```python
from build123d import *

# Parameters (mm, degrees)
SKETCH1_R           = 53.975
SKETCH1_R_2         = 3.302
BOSS_EXTRUDE1_DEPTH = 3.175
SKETCH2_R           = 28.575
BOSS_EXTRUDE2_DEPTH = 136.525
SKETCH3_W           = 40.450959828
SKETCH3_H           = 34.29
CUT_EXTRUDE1_DEPTH  = 136.525
SKETCH4_W           = 24.671855952
SKETCH4_H           = 34.29
CUT_EXTRUDE2_DEPTH  = 49.53
FILLET1_R           = 2.54


with BuildPart() as part:
    # Sketch1 → Boss-Extrude1 (new body)
    with BuildSketch(Plane(origin=(0, 0, 0), x_dir=(1, 0, 0), z_dir=(0, 1, 0))):
        with Locations(Location((0, 0, 0), (0, 0, 270))):
            Circle(SKETCH1_R)
        with Locations(Location((0, 47.625, 0), (0, 0, 270))):
            Circle(SKETCH1_R_2, mode=Mode.SUBTRACT)
        with Locations(Location((45.294066589, 14.716934357, 0), (0, 0, 270))):
            Circle(SKETCH1_R_2, mode=Mode.SUBTRACT)
        with Locations(Location((27.99327264, -38.529434357, 0), (0, 0, 270))):
            Circle(SKETCH1_R_2, mode=Mode.SUBTRACT)
        with Locations(Location((-27.99327264, -38.529434357, 0), (0, 0, 270))):
            Circle(SKETCH1_R_2, mode=Mode.SUBTRACT)
        with Locations(Location((-45.294066589, 14.716934357, 0), (0, 0, 270))):
            Circle(SKETCH1_R_2, mode=Mode.SUBTRACT)
    extrude(amount=BOSS_EXTRUDE1_DEPTH)

    # Sketch2 → Boss-Extrude2 (add)
    with BuildSketch(Plane(origin=(0, 3.175, 0), x_dir=(1, 0, 0), z_dir=(0, 1, 0))):
        with Locations(Location((0, 0, 0), (0, 0, 270))):
            Circle(SKETCH2_R)
    extrude(amount=BOSS_EXTRUDE2_DEPTH)

    # Sketch3 → Cut-Extrude1 (cut)
    with BuildSketch(Plane(origin=(0, 139.7, 0), x_dir=(1, 0, 0), z_dir=(0, 1, 0))):
        with Locations((43.085479914, 0)):
            Rectangle(SKETCH3_W, SKETCH3_H)
    extrude(amount=-CUT_EXTRUDE1_DEPTH, mode=Mode.SUBTRACT)

    # Sketch4 → Cut-Extrude2 (cut)
    with BuildSketch(Plane(origin=(0, 3.175, 0), x_dir=(1, 0, 0), z_dir=(0, 1, 0))):
        with Locations((-35.195927976, 0)):
            Rectangle(SKETCH4_W, SKETCH4_H)
    extrude(amount=CUT_EXTRUDE2_DEPTH, mode=Mode.SUBTRACT)

    # Fillet1
    fillet1_edges = [part.edges().sort_by_distance(p)[0] for p in [
        (-28.575, 139.7, 0),
        (22.86, 139.7, 0),
        (22.86, 71.4375, 17.145),
        (22.86, 71.4375, -17.145),
        (-28.575, 52.705, 0),
        (-22.86, 27.94, 17.145),
        (-22.86, 27.94, -17.145),
    ]]
    fillet(fillet1_edges, radius=FILLET1_R)
    fillet1_2_edges = [part.edges().sort_by_distance(p)[0] for p in [
        (0, 3.175, -28.575),
        (22.86, 3.175, 0),
        (0, 3.175, 28.575),
        (-22.86, 3.175, 0),
        (-22.716559526, 3.175, -17.117815364),
        (-22.716559526, 3.175, 17.117815364),
        (22.716559526, 3.175, 17.117815364),
        (22.716559526, 3.175, -17.117815364),
    ]]
    fillet(fillet1_2_edges, radius=FILLET1_R)


solid = part.part
```
Geometry: final body of the model. Coordinates: model frame, mm. A direction names the side the tool comes from. Coordinates: 2 decimals unless noted, no trailing zeros. Order: outer loops, then holes, each group sorted by start corner. A loop starts at its lowest first (then second) coordinate and runs counter-clockwise, first axis right, second up. Notation, with made-up numbers: (22.5, 24) -> (73.5, 24) arc R28 ccw to (73.5, 58) -> close; hole circle Ø6 at (43.5, -39.75). An arc over 180 degrees is marked (long way). Write item = value, one per line.
(1) Cut plane A-A on x = 0. Return loops of the section in (y, z) (3 decimals).
Solved:
outline = (0, -53.975) -> (3.175, -53.975) -> (3.175, -50.927) -> (0, -50.927) -> close; (0, -44.323) -> (3.175, -44.323) -> (3.175, -31.115) arc R2.54 cw to (5.715, -28.575) -> (137.16, -28.575) arc R2.54 ccw to (139.7, -26.035) -> (139.7, 26.035) arc R2.54 ccw to (137.16, 28.575) -> (5.715, 28.575) arc R2.54 cw to (3.175, 31.115) -> (3.175, 53.975) -> (0, 53.975) -> close
(2) Cut plane D-D on y = 107. Return loops of the section in (x, z) (3 decimals), plus the area to 3 significant figures.
Solved:
outline = (22.302, -17.864) arc R2.54 ccw to (22.86, -16.276) -> (22.86, 16.276) arc R2.54 ccw to (22.302, 17.864) arc R28.575 ccw (long way) to start
area = 2,430 mm²
(3) Cut plane B-B on y = 38. Return loops of the section in (x, z) (3 decimals), plus the area to 3 significant figures.
Solved:
outline = (-22.86, -16.276) arc R2.54 ccw to (-22.302, -17.864) arc R28.575 ccw to (22.302, -17.864) arc R2.54 ccw to (22.86, -16.276) -> (22.86, 16.276) arc R2.54 ccw to (22.302, 17.864) arc R28.575 ccw to (-22.302, 17.864) arc R2.54 ccw to (-22.86, 16.276) -> close
area = 2,300 mm²
(4) Pull-direction query (X, two-part tool) for faces 1 (the cylindrical face through (0.145, 1.565, -50.924)), 2 (the flat face through (22.86, 72, 0)), 3 (the cylindrical face through (-28.558, 70.517, -0.986)); classes: pulls with the +X half, pulls with the -X half, needs draft (parallel to the pull), parting line crosses it, or undercut.
Solved:
face_1 = undercut
face_2 = pulls with the +X half
face_3 = parting line crosses it
(5) Line query: line 1 (Y direction, x = 41.5, z = 19) (3 decimals); line 2 (X direction, y = 50, z = -9); line 3 (Z direction, x = 3.5, y = 33.5). Output: solid intervals per line, ascending.
Solved:
line_1 = 0 to 3.175
line_2 = -22.86 to 22.86
line_3 = -28.36 to 28.36
(6) Pin query (flat end, axial travel): pin 1 Ø12 at (y, z) = (111, -32) entering from +X; pin 2 Ø3 at (x, y) = (-6, 51.5) entering from +Z; pin 3 Ø7.5 at (x, z) = (45.29, -14.72) entering from +Y (3 decimals). Return the tip coordinate at first contact, or that it passes through.
Solved:
pin_1 = 11.85
pin_2 = 28.22
pin_3 = 3.175
(7) Cut plane C-C on z = 0. Return loops of the section in (x, y) (3 decimals), plus the area to 3 significant figures.
Solved:
outline = (-53.975, 0) -> (53.975, 0) -> (53.975, 3.175) -> (25.4, 3.175) arc R2.54 cw to (22.86, 5.715) -> (22.86, 137.16) arc R2.54 ccw to (20.32, 139.7) -> (-26.035, 139.7) arc R2.54 ccw to (-28.575, 137.16) -> (-28.575, 55.245) arc R2.54 ccw to (-26.035, 52.705) -> (-22.86, 52.705) -> (-22.86, 5.715) arc R2.54 cw to (-25.4, 3.175) -> (-53.975, 3.175) -> close
area = 7,080 mm²
(8) Access query for faces 4 (the flat face through (-22.86, 29, 0)), 5 (the cylindrical face through (28.14, 1.57, 35.23)). Directions: +Z, -Z, +X, -X, +Y, -Y. A direction counts if a zero-diameter tool reaches every point of the face in a straight line with its end or side. Return the directions, or none.
Solved:
face_4 = +Z, -Z, -X
face_5 = +Y, -Y
